from build123d import *

# Parameters (mm, degrees)
F0_W     = 5
F0_H     = 5
F2_D     = 3
F2_DEPTH = 100.001
F3_D     = 3


with BuildPart() as f1:
    # F0 (on Right) → F1 (revolve)
    with BuildSketch(Plane.YZ):
        with Locations((-97.5, 2.3040431552)):
            Rectangle(F0_W, F0_H)
    revolve(axis=Axis((0, 0, 1.25), (0, 0, -1)))

    # F2 (through all, one way)
    with BuildSketch(Plane.YZ):
        with Locations((0, 2.5)):
            Circle(F2_D / 2)
    extrude(amount=-F2_DEPTH, mode=Mode.SUBTRACT)

    # F3 (through all)
    with Locations(Plane(origin=(0, 0, 0), x_dir=(0, 1, 0), z_dir=(-1, 0, 0))):
        with Locations((0, -2.5)):
            Hole(F3_D / 2)


solid = f1.part
Check sheet for the modelled part. Datum: model origin and axes. Units: mm. Give positions to 0.01 mm unless a question says otherwise; leave off trailing zeros. Write each loop counter-clockwise with the first axis right and the second up, starting at its lowest first coordinate (ties: lowest second). Pieces come first, ordered by that corner, then holes. Notation, with made-up numbers: (71.25, 23.25) -> (118.25, 23.25) arc R20 cw to (118.25, 49.25) -> close; hole circle Ø4 at (65.5, -17.75). An arc over 180 degrees is marked (long way). Use one line per item in the form item = value. Start each with the question number.
1. Mould release check, pull along X, two halves, no side actions. Record for faces 1 (the flat face through (37, -88, -0.196)), 2 (the cylindrical face through (-30.04, -95.38, 2.34)), 3 (the cylindrical face through (92.74, 20.59, 2.34)): pulls with the +X half, pulls with the -X half, needs draft (parallel to the pull), parting line crosses it, or undercut.
2. Section check B-B (y = -28). Record the cut outline in (x, z), and give its area (3 significant figures).
3. Thickness scan on line 1 along Z through (x, y) = (-96.75, 0); line 2 along X through (y, z) = (-19, 4.3); line 3 along X through (y, z) = (-80.5, 4). Record the ranges inside material, lowest first. Write a range as from..to.
4. Section check A-A (x = 0). Record the cut outline in (y, z), and give its area (3 significant figures).
5. Go/stop test with a flat-tipped pin: P1, Ø2, axis at y = -76, z = 2, coming from the +X side. Record where the tip stops, or that it passes through.
Conclusion:
q1.face_1 = needs draft
q1.face_2 = parting line crosses it
q1.face_3 = undercut
q2.outline = (-96, -0.2) -> (-90.78, -0.2) -> (-90.78, 4.8) -> (-96, 4.8) -> close; (90.78, -0.2) -> (96, -0.2) -> (96, 4.8) -> (90.78, 4.8) -> close
q2.area = 52.2 mm²
q3.line_1 = -0.2..1, 4..4.8
q3.line_2 = -98.18..-93.08, 93.08..98.18
q3.line_3 = -59.33..-50.45, 50.45..59.33
q4.outline = (-100, -0.2) -> (-95, -0.2) -> (-95, 4.8) -> (-100, 4.8) -> close; (95, -0.2) -> (100, -0.2) -> (100, 4.8) -> (95, 4.8) -> close
q4.area = 50.0 mm²
q5.P1 = 66.14
